Work out the finished part from the listing and answer in its coordinate system (mm). A direction names the side the tool comes from. Round coordinates to 2 decimals unless told otherwise and drop trailing zeros. Order: outer loops, then holes, each group sorted by start corner. A loop starts at its lowest first (then second) coordinate and runs counter-clockwise, first axis right, second up. Notation, with made-up numbers: M -0.75,59 L 26.25,59 A27 ccw 26.25,95 Z; hole C -8.5,18 d9. An arc over 180 degrees is marked long. Return JSON: item names as keys, results as strings.
from build123d import *

# Parameters (mm, degrees)
SKETCH_1_W          = 7
SKETCH_1_H          = 4
EXTRUDE_1_DEPTH     = 1.3
SKETCH_2_W          = 1.3
SKETCH_2_H          = 4
EXTRUDE_2_DEPTH     = 11
SKETCH_3_R          = 1
CUT_EXTRUDE_1_DEPTH = 2
SKETCH_4_R          = 1
CUT_EXTRUDE_2_DEPTH = 7


with BuildPart() as part:
    # 草图1 → 凸台-拉伸1 (new body)
    with BuildSketch(Plane.XY):
        with Locations((3.5, 2)):
            Rectangle(SKETCH_1_W, SKETCH_1_H)
    extrude(amount=EXTRUDE_1_DEPTH)

    # 草图2 → 凸台-拉伸2 (add)
    with BuildSketch(Plane.XY.offset(1.3)):
        with Locations((0.65, 2)):
            Rectangle(SKETCH_2_W, SKETCH_2_H)
        with Locations((6.35, 2)):
            Rectangle(SKETCH_2_W, SKETCH_2_H)
    extrude(amount=EXTRUDE_2_DEPTH)

    # 草图3 → 切除-拉伸1 (cut)
    with BuildSketch(Plane.XY.offset(1.3)):
        with Locations((3.5, 2)):
            Circle(SKETCH_3_R)
    extrude(amount=-CUT_EXTRUDE_1_DEPTH, mode=Mode.SUBTRACT)

    # 草图4 → 切除-拉伸2 (cut)
    with BuildSketch(Plane(origin=(7, 0, 0), x_dir=(0, 0, -1), z_dir=(1, 0, 0))):
        with Locations((-10.4, 2)):
            Circle(SKETCH_4_R)
    extrude(amount=-CUT_EXTRUDE_2_DEPTH, mode=Mode.SUBTRACT)


solid = part.part
Item 1: Find section A-A (x = 3.5). Determine the outline of the cut face in (y, z), plus the area to 3 significant figures.
Output:
{"outline": "M 0,0 L 1,0 L 1,1.3 L 0,1.3 Z; M 3,0 L 4,0 L 4,1.3 L 3,1.3 Z", "area": "2.60 mm^2"}
Item 2: Find section D-D (z = 10.4). Determine the outline of the cut face in (x, y), plus the area to 3 significant figures.
Output:
{"outline": "M 0,0 L 1.3,0 L 1.3,1 L 0,1 Z; M 0,3 L 1.3,3 L 1.3,4 L 0,4 Z; M 5.7,0 L 7,0 L 7,1 L 5.7,1 Z; M 5.7,3 L 7,3 L 7,4 L 5.7,4 Z", "area": "5.20 mm^2"}
Item 3: This flat-tipped pin is pushed along its axis until it touches: pin 1 (2 mm diameter, centred on y = 3, z = 9, fed in from -X). Where does it stop, or does it pass through?
Output:
{"pin 1": "stops at x = 0"}
Item 4: Find section C-C (z = 6.75). Determine the outline of the cut face in (x, y), plus the area to 3 significant figures.
Output:
{"outline": "M 0,0 L 1.3,0 L 1.3,4 L 0,4 Z; M 5.7,0 L 7,0 L 7,4 L 5.7,4 Z", "area": "10.4 mm^2"}
Item 5: The mould has two halves that part along Z. Classify faces 1 (the flat face through (2.7, 1.1, 0)), 2 (the cylindrical face through (6.359, 1.617, 9.476)), 3 (the cylindrical face through (0.659, 1.617, 9.476)), 4 (the flat face through (7, 2, 6)): pulls with the +Z half, pulls with the -Z half, needs draft (parallel to the pull), parting line crosses it, or undercut.
Output:
{"face 1": "pulls with the -Z half", "face 2": "undercut", "face 3": "undercut", "face 4": "needs draft"}
Item 6: Consider line 1 along X through (y, z) = (1.4, 11.25); line 2 along Y through (x, z) = (6.45, 10.4); line 3 along Z through (x, y) = (2, 3). Determine where each line is inside the solid, lowest interval first. Write a range as [from, to].
Output:
{"line 1": "x = [0, 1.3], [5.7, 7]", "line 2": "y = [0, 1], [3, 4]", "line 3": "z = [0, 1.3]"}
Item 7: Find section B-B (y = 2). Determine the outline of the cut face in (x, z).
Output:
{"outline": "M 0,0 L 2.5,0 L 2.5,1.3 L 1.3,1.3 L 1.3,9.4 L 0,9.4 Z; M 0,11.4 L 1.3,11.4 L 1.3,12.3 L 0,12.3 Z; M 4.5,0 L 7,0 L 7,9.4 L 5.7,9.4 L 5.7,1.3 L 4.5,1.3 Z; M 5.7,11.4 L 7,11.4 L 7,12.3 L 5.7,12.3 Z"}
Item 8: Which of the six approach directions +Z, -Z, +X, -X, +Y, -Y give full straight-line access (tool end or side, diameter ignored) to faces 5 (the flat face through (2, 2, 1.3)), 6 (the flat face through (6, 2, 12.3))?
Output:
{"face 5": "+Z, +Y, -Y", "face 6": "+Z, +X, -X, +Y, -Y"}
